Model file for the job. Use its own axes, mm. Face numbers are marked on the shaded views. A direction names the side the tool comes from. Coordinates: 2 decimals unless noted, no trailing zeros. Order: outer loops, then holes, each group sorted by start corner. A loop starts at its lowest first (then second) coordinate and runs counter-clockwise, first axis right, second up. Notation, with made-up numbers: (23, 85.5) -> (42, 85.5) arc R23 cw to (42, 96.5) -> close; hole circle Ø3 at (0, -14). An arc over 180 degrees is marked (long way). Write item = value, one per line. Start each with the question number.
Q1. Cut at A-A, the plane x = 0. List the corners of the cut face in (y, z) (3 decimals).
Q2. Mould opens along X. For the marked faces 1, 2 and 3 say: +X half, -X half, draft (parallel to the pull), parting line (faces both ways), or undercut.
Q3. Cut at D-D, the plane z = -9.5. List the corners of the cut face in (x, y) (3 decimals).
Q4. Cut at B-B, the plane z = 0. List the corners of the cut face in (x, y) (3 decimals).
Q5. Wall check: line 1 (Z direction, x = 1.75, y = 2.4); line 2 (Z direction, x = 2.25, y = 1.45); line 3 (X direction, y = 1.1, z = 8.75). Give the ranges that are in metal, low to high. Write a range as from..to.
Q6. Cut at C-C, the plane y = 0.9. List the corners of the cut face in (x, z) (3 decimals).
Q7. 3-axis set-ups, long thin cutter, end or side, ignore diameter. For the marked faces 4 and 5: which of +Z, -Z, +X, -X, +Y, -Y reach the whole face in a straight line?
from build123d import *

# Parameters (mm, degrees)
SKETCH1_R           = 12.7
BOSS_EXTRUDE1_DEPTH = 3.175


with BuildPart() as part:
    # Sketch1 → Boss-Extrude1 (new body)
    with BuildSketch(Plane(origin=(0, 0, 0), x_dir=(1, 0, 0), z_dir=(0, 1, 0))):
        Circle(SKETCH1_R)
        with BuildLine():
            Line((-1.725, 1.945347013), (1.725, 1.945347013))
            ThreePointArc((1.725, 1.945347013), (2.592456696, -0.197909772), (1.409713207, -2.184652987))
            Line((1.409713207, -2.184652987), (-1.409713207, -2.184652987))
            ThreePointArc((-1.409713207, -2.184652987), (-2.592456696, -0.197909772), (-1.725, 1.945347013))
        make_face(mode=Mode.SUBTRACT)
    extrude(amount=BOSS_EXTRUDE1_DEPTH)


solid = part.part
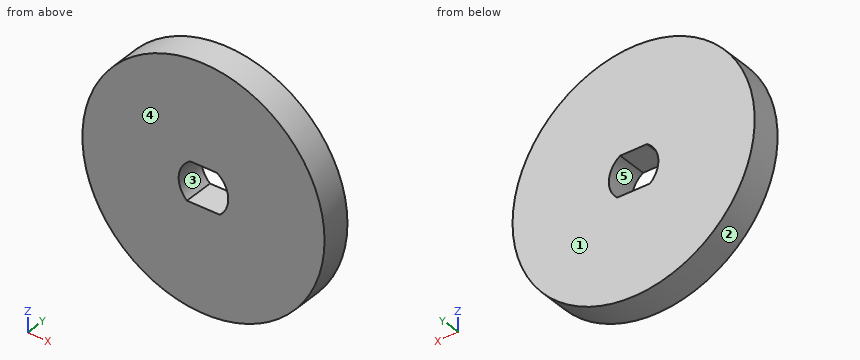
Here are the results:
q1.outline = (0, -12.7) -> (3.175, -12.7) -> (3.175, -1.945) -> (0, -1.945) -> close; (0, 2.185) -> (3.175, 2.185) -> (3.175, 12.7) -> (0, 12.7) -> close
q2.face_1 = draft
q2.face_2 = parting line
q2.face_3 = undercut
q3.outline = (-8.429, 0) -> (8.429, 0) -> (8.429, 3.175) -> (-8.429, 3.175) -> close
q4.outline = (-12.7, 0) -> (-2.6, 0) -> (-2.6, 3.175) -> (-12.7, 3.175) -> close; (2.6, 0) -> (12.7, 0) -> (12.7, 3.175) -> (2.6, 3.175) -> close
q5.line_1 = -12.58..-1.92, 1.92..12.58
q5.line_2 = -12.5..-1.3, 1.3..12.5
q5.line_3 = -9.2..9.2
q6.outline = circle Ø25.4 at (0, 0); hole (-1.725, -1.945) -> (1.725, -1.945) arc R2.6 ccw to (1.41, 2.185) -> (-1.41, 2.185) arc R2.6 ccw to start
q7.face_4 = +Z, -Z, +X, -X, -Y
q7.face_5 = +Y, -Y
